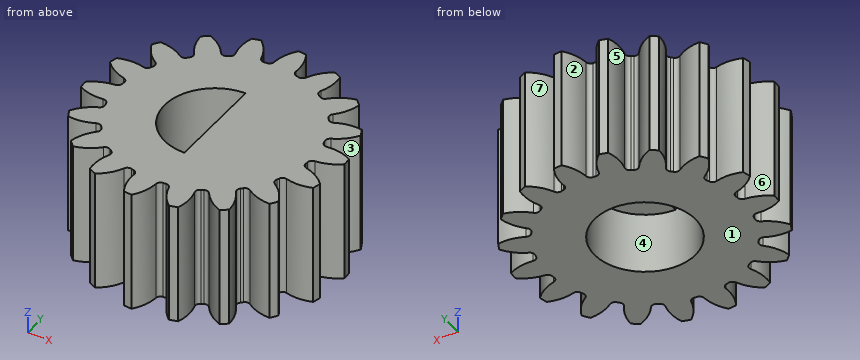
from build123d import *

# Parameters (mm, degrees)
SKETCH3_R           = 7.9375
GEARBODY_DEPTH      = 7.62
TOOTHCUT_DEPTH      = 8.62
CIRPATTERN1_COUNT   = 18
BOREDIA_R           = 3.175
BORE_DEPTH          = 12700
BOSS_EXTRUDE1_DEPTH = 3.81


with BuildPart() as part:
    # Sketch3 → gearBody (new body)
    with BuildSketch(Plane.XY):
        Circle(SKETCH3_R)
    extrude(amount=GEARBODY_DEPTH)

    # Sketch2 → toothCut (cut, through all)
    with BuildSketch(Plane.XY):
        with BuildLine():
            ThreePointArc((6.109024448, -0.620440562), (6.116845087, -0.537896263), (6.123550449, -0.45525389))
            ThreePointArc((6.123550449, -0.45525389), (6.211734547, -0.262957543), (6.404089586, -0.174901543))
            ThreePointArc((6.404089586, -0.174901543), (7.575851051, 0.185269566), (8.474852534, 1.018662927))
            ThreePointArc((8.474852534, 1.018662927), (8.503040528, -0.747730842), (8.167006715, -2.482096081))
            ThreePointArc((8.167006715, -2.482096081), (7.427249601, -1.504595405), (6.336329857, -0.945451173))
            ThreePointArc((6.336329857, -0.945451173), (6.162294814, -0.825175973), (6.109024448, -0.620440562))
        make_face()
    toothcut = extrude(amount=TOOTHCUT_DEPTH, mode=Mode.SUBTRACT)

    # CirPattern1: toothCut ×18 about axis
    cirpattern1_axis = Axis((0, 0, 0), (0, 0, 1))
    for i in range(1, CIRPATTERN1_COUNT):
        add(toothcut.rotate(cirpattern1_axis, i * 360 / CIRPATTERN1_COUNT), mode=Mode.SUBTRACT)

    # boreDia → bore (cut, symmetric)
    with BuildSketch(Plane.XY):
        Circle(BOREDIA_R)
    extrude(amount=BORE_DEPTH, both=True, mode=Mode.SUBTRACT)

    # Sketch5 → Boss-Extrude1 (add)
    with BuildSketch(Plane.XY.offset(7.62)):
        with BuildLine():
            Line((0, 3.175), (0, -3.175))
            ThreePointArc((0, -3.175), (3.175, 0), (0, 3.175))
        make_face()
    extrude(amount=-BOSS_EXTRUDE1_DEPTH)


solid = part.part
Verification items for the finished model (mm, model axes). Face numbers are marked on the shaded views. A direction names the side the tool comes from. Coordinates: 2 decimals unless noted, no trailing zeros. Use a Markdown table: item, result.
Q1. Go/stop test with flat-tipped pins: P1, Ø2, axis at x = 3.5, z = 4, coming from the +Y side; P2, Ø2, axis at x = -2.5, z = 5.5, coming from the -Y side; P3, Ø3.5, axis at x = 2, y = 0.5, coming from the -Z side; P4, Ø3, axis at y = 1.5, z = 5, coming from the -X side. Record where each tip stops, or that it passes through.
Reply:
| item | result |
|---|---|
| P1 | stops at y = 7.3 |
| P2 | stops at y = -7.3 |
| P3 | stops at z = 0 |
| P4 | stops at x = -7.73 |
Q2. Set-up check for the marked faces 4, 5, 6 and 7: record each of +Z, -Z, +X, -X, +Y, -Y from which the full face is reachable in a straight line by a thin tool's end or side.
Reply:
| item | result |
|---|---|
| face 4 | -Z |
| face 5 | +Z, -Z |
| face 6 | +Z, -Z, -X |
| face 7 | +Z, -Z, +Y |
Q3. Thickness scan on line 1 (X direction, y = -7, z = 4.75); line 2 (X direction, y = 7, z = 6.5); line 3 (X direction, y = -6.5, z = 2). Record the ranges inside material, lowest first.
Reply:
| item | result |
|---|---|
| line 1 | x = -3.61 to -2.71, -1.26 to 0.06, 1.2 to 2.44 |
| line 2 | x = -2.44 to -1.2, -0.06 to 1.26, 2.71 to 3.61 |
| line 3 | x = -3.62 to -2.27, -1.3 to 0.16, 0.99 to 2.44, 4 to 4.56 |
Q4. Draft check along X on the marked faces 1, 2 and 3. Enter one of: +X half, -X half, draft (parallel to the pull), parting line (faces both ways), or undercut.
Reply:
| item | result |
|---|---|
| face 1 | draft |
| face 2 | undercut |
| face 3 | +X half |
